Study the drawing (mm; zero at the part's minimum x, y, z) and answer. A direction names the side the tool comes from. Round coordinates to 2 decimals unless told otherwise and drop trailing zeros. Write each loop counter-clockwise with the first axis right and the second up, starting at its lowest first coordinate (ties: lowest second). Pieces come first, ordered by that corner, then holes. Notation, with made-up numbers: M 0.5,27 L 59.5,27 A28 cw 59.5,57 Z; hole C -26.5,82 d3. An arc over 180 degrees is marked long. Put each result on its own line as item: value. Start each with the question number.
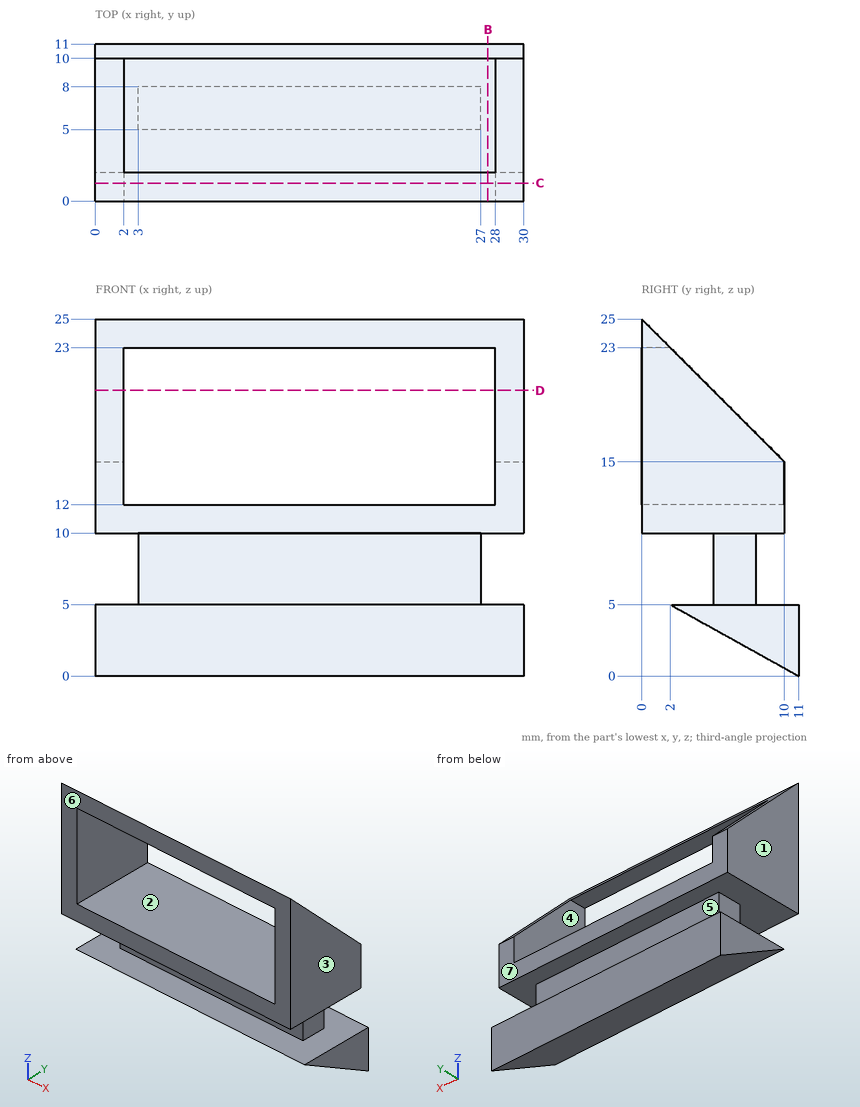
Item 1: Flat-ended cylindrical pins translate along their axes: pin 1 (1.5 mm diameter, centred on x = 17.5, z = 13, fed in from +Y); pin 2 (4 mm diameter, centred on x = 14, z = 7.5, fed in from -Y); pin 3 (0.6 mm diameter, centred on x = 11.5, y = 0.5, fed in from -Z); pin 4 (1 mm diameter, centred on x = 15, y = 3.5, fed in from -Z). Find the tip coordinate at first contact, or state that the pin passes through.
Item 2: Section D-D (z = 20) is taken. Give the vertices of the cut face in (x, y), and give its area (3 significant figures).
Item 3: Determine the mould class of the marked faces 1, 2 and 3 for opening direction X: released by +X, released by -X, zero draft, split by the parting line, or undercut.
Item 4: Consider line 1 along X through (y, z) = (3, 12.5); line 2 along Z through (x, y) = (13, 0.75); line 3 along Z through (x, y) = (6, 1). Determine where each line is inside the solid, lowest interval first. Write a range as [from, to].
Item 5: Section C-C (y = 1.25) is taken. Give the vertices of the cut face in (x, z), and give its area (4 significant figures).
Item 6: Which of the six approach directions +Z, -Z, +X, -X, +Y, -Y give full straight-line access (tool end or side, diameter ignored) to the marked faces 4, 5, 6 and 7?
Item 7: Section B-B (x = 27.5) is taken. Count the separate pieces of the cut face and the enclosed holes in it, and give its area (3 significant figures).
Output values:
1. pin 1: passes through
1. pin 2: stops at y = 5
1. pin 3: stops at z = 10
1. pin 4: stops at z = 3.89
2. outline: M 0,0 L 2,0 L 2,5 L 0,5 Z; M 28,0 L 30,0 L 30,5 L 28,5 Z
2. area: 20.0 mm^2
3. face 1: released by -X
3. face 2: undercut
3. face 3: released by +X
4. line 1: x = [0, 2], [28, 30]
4. line 2: z = [10, 12], [23, 24.25]
4. line 3: z = [10, 12], [23, 24]
5. outline: M 0,10 L 30,10 L 30,23.75 L 0,23.75 Z; hole M 2,12 L 28,12 L 28,23 L 2,23 Z
5. area: 126.5 mm^2
6. face 4: +Y, -Y
6. face 5: +X, -X, +Y
6. face 6: +Z, -Z, +X, -X, -Y
6. face 7: +Z, +X, -X, +Y
7. separate pieces: 3
7. enclosed holes: 0
7. area: 44.5 mm^2
